Can you work these out from the model? Positions are in its coordinate system, mm. Face numbers are marked on the shaded views. A direction names the side the tool comes from. Round coordinates to 2 decimals unless told otherwise and drop trailing zeros. Loops run counter-clockwise (first coordinate to the right, second up) from the corner with the lowest first, then second, coordinate; pieces in that order, holes last. Notation, with made-up numbers: M -27,20.5 L -4,20.5 A6 cw -4,25.5 Z; hole C -25.75,-31.75 d9. An arc over 180 degrees is marked long. Return JSON: item names as keys, results as strings.
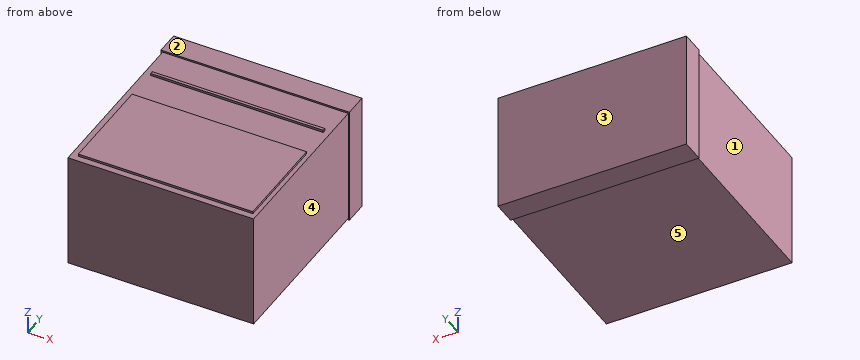
```python
from build123d import *

# Parameters (mm, degrees)
SKETCH_W      = 800
SKETCH_H      = 500
PAD_DEPTH     = 850
SKETCH001_W   = 812.236467
SKETCH001_H   = 514.082147
PAD001_DEPTH  = 100
SKETCH002_W   = 743.373808
SKETCH002_H   = 12.635254
SKETCH002_W_2 = 751.797392
SKETCH002_H_2 = 425.38678
PAD002_DEPTH  = 10


with BuildPart() as part:
    # Sketch → Pad (new body)
    with BuildSketch(Plane.XZ):
        with Locations((400, 250)):
            Rectangle(SKETCH_W, SKETCH_H)
    extrude(amount=PAD_DEPTH)

    # Sketch001 (on Face5 of Pad) → Pad001 (join)
    with BuildSketch(Plane(origin=(0, 0, 0), x_dir=(1, 0, 0), z_dir=(0, 1, 0))):
        with Locations((398.720084, -250.168399)):
            Rectangle(SKETCH001_W, SKETCH001_H)
    extrude(amount=-PAD001_DEPTH)

    # Sketch002 (on Face8 of Pad001) → Pad002 (join)
    with BuildSketch(Plane(origin=(0, 0, 500), x_dir=(-1, 0, 0), z_dir=(0, 0, 1))):
        with Locations((-401.667527, 243.347824)):
            Rectangle(SKETCH002_W, SKETCH002_H)
        with Locations((-405.879319, 609.770111)):
            Rectangle(SKETCH002_W_2, SKETCH002_H_2)
    extrude(amount=PAD002_DEPTH)


solid = part.part
```
Q1. Suppose I cut it at C-C, the plane y = -189.5. Please give me the cut outline in (x, z), plus the area to 3 significant figures.
Results:
{"outline": "M 0,0 L 800,0 L 800,500 L 0,500 Z", "area": "400,000 mm2"}
Q2. Suppose I cut it at B-B, the plane x = 293.5. Please give me the cut outline in (y, z), plus the area to 3 significant figures.
Results:
{"outline": "M -850,0 L -100,0 L -100,-6.87 L 0,-6.87 L 0,507.21 L -100,507.21 L -100,500 L -237.03,500 L -237.03,510 L -249.67,510 L -249.67,500 L -397.08,500 L -397.08,510 L -822.46,510 L -822.46,500 L -850,500 Z", "area": "431,000 mm2"}
Q3. On a 3-axis mill with a long thin cutter (end or side, diameter ignored), from which of +Z, -Z, +X, -X, +Y, -Y can I reach the whole of each face in a straight line? I mean the marked faces 1, 2, 3, 4 and 5. Say none if no direction works.
Results:
{"face 1": "+Z, -Z, -X, -Y", "face 2": "+Z, +X, -X, +Y", "face 3": "+Z, -Z, +X, -X, +Y", "face 4": "+Z, -Z, +X, -Y", "face 5": "-Z, +X, -X, -Y"}
Q4. Suppose I cut it at A-A, the plane y = -769.5. Please give me the cut outline in (x, z).
Results:
{"outline": "M 0,0 L 800,0 L 800,500 L 781.78,500 L 781.78,510 L 29.98,510 L 29.98,500 L 0,500 Z"}
Q5. If I drill on line 1 along Z through (x, y) = (377.5, -115); line 2 along Z through (x, y) = (129, -677.5); line 3 along X through (y, z) = (-771.5, 459.5), over which ranges is the centre line in solid material (lowest first)?
Results:
{"line 1": "z = 0 to 500", "line 2": "z = 0 to 510", "line 3": "x = 0 to 800"}
Q6. I'm going to push flat-ended pins straight in: pin 1 Ø4 at (x, y) = (86.5, -180.5) entering from -Z; pin 2 Ø2 at (y, z) = (-590.5, 416.5) entering from +X; pin 3 Ø1 at (y, z) = (-423.5, 240.5) entering from -X. Where does each tip first touch, or does it pass through?
Results:
{"pin 1": "stops at z = 0", "pin 2": "stops at x = 800", "pin 3": "stops at x = 0"}
